```python
from build123d import *

# Parameters (mm, degrees)
SKETCH1_W           = 120
SKETCH1_H           = 140
BOSS_EXTRUDE1_DEPTH = 3
SKETCH2_R           = 1.525
CUT_EXTRUDE1_DEPTH  = 93.244241013
SKETCH3_W           = 10
SKETCH3_H           = 2.05
CUT_EXTRUDE2_DEPTH  = 93.244241013
SKETCH4_R           = 1.5
CUT_EXTRUDE3_DEPTH  = 3
SKETCH5_R           = 1.5
SKETCH5_W           = 50
SKETCH5_H           = 8
CUT_EXTRUDE4_DEPTH  = 3


with BuildPart() as part:
    # Sketch1 → Boss-Extrude1 (new body)
    with BuildSketch(Plane(origin=(0, 0, 0), x_dir=(1, 0, 0), z_dir=(0, 1, 0))):
        Rectangle(SKETCH1_W, SKETCH1_H)
    extrude(amount=BOSS_EXTRUDE1_DEPTH)

    # Sketch2 → Cut-Extrude1 (cut, through all)
    with BuildSketch(Plane(origin=(0, 3, 0), x_dir=(1, 0, 0), z_dir=(0, 1, 0))):
        with Locations(Location((-53, -26.81, 0), (0, 0, 270))):
            Circle(SKETCH2_R)
        with Locations(Location((-54, 60, 0), (0, 0, 270))):
            Circle(SKETCH2_R)
        with Locations(Location((53, -26.81, 0), (0, 0, 90))):
            Circle(SKETCH2_R)
        with Locations(Location((54, 60, 0), (0, 0, 90))):
            Circle(SKETCH2_R)
    extrude(amount=-CUT_EXTRUDE1_DEPTH, mode=Mode.SUBTRACT)

    # Sketch3 → Cut-Extrude2 (cut, through all)
    with BuildSketch(Plane(origin=(0, 3, 0), x_dir=(1, 0, 0), z_dir=(0, 1, 0))):
        with Locations((0, 16.115)):
            Rectangle(SKETCH3_W, SKETCH3_H)
        with Locations((0, -15.985)):
            Rectangle(SKETCH3_W, SKETCH3_H)
        with Locations((0, 61.215)):
            Rectangle(SKETCH3_W, SKETCH3_H)
    extrude(amount=-CUT_EXTRUDE2_DEPTH, mode=Mode.SUBTRACT)

    # Sketch4 → Cut-Extrude3 (cut)
    with BuildSketch(Plane(origin=(0, 3, 0), x_dir=(1, 0, 0), z_dir=(0, 1, 0))):
        with Locations(Location((-52, -50, 0), (0, 0, 270))):
            Circle(SKETCH4_R)
        with Locations(Location((-45.815341562, -62, 0), (0, 0, 270))):
            Circle(SKETCH4_R)
        with Locations(Location((45.815341562, -62, 0), (0, 0, 90))):
            Circle(SKETCH4_R)
        with Locations(Location((52, -50, 0), (0, 0, 90))):
            Circle(SKETCH4_R)
    extrude(amount=-CUT_EXTRUDE3_DEPTH, mode=Mode.SUBTRACT)

    # Sketch5 → Cut-Extrude4 (cut)
    with BuildSketch(Plane(origin=(0, 3, 0), x_dir=(1, 0, 0), z_dir=(0, 1, 0))):
        with Locations(Location((-36.8, -65, 0), (0, 0, 270))):
            Circle(SKETCH5_R)
        with Locations(Location((36.8, -65, 0), (0, 0, 90))):
            Circle(SKETCH5_R)
        with Locations((0, -55.5)):
            Rectangle(SKETCH5_W, SKETCH5_H)
    extrude(amount=-CUT_EXTRUDE4_DEPTH, mode=Mode.SUBTRACT)


solid = part.part
```
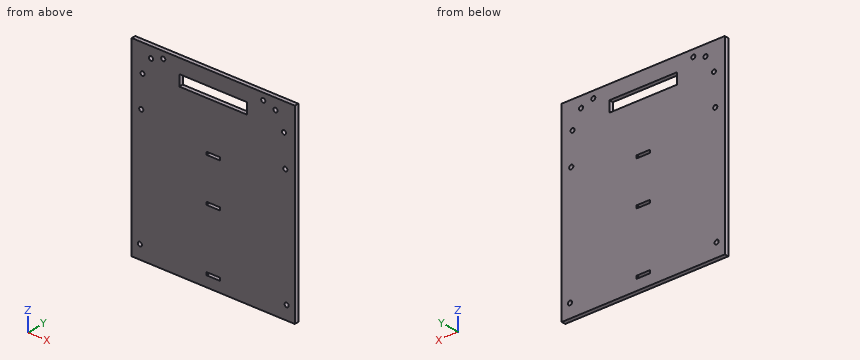
CAD build for the part. Positions are in the model's coordinates, mm. Round coordinates to 2 decimals unless told otherwise and drop trailing zeros. Write each loop counter-clockwise with the first axis right and the second up, starting at its lowest first coordinate (ties: lowest second). Pieces come first, ordered by that corner, then holes. Notation, with made-up numbers: (18.5, 61) -> (72.5, 61) arc R9 cw to (72.5, 68) -> close; hole circle Ø2 at (6.25, -25.75). An arc over 180 degrees is marked (long way). Answer in a Markdown table with one row per item. Add a question column.
Item 1: Saw through at A-A, the plane z = 62. Write the cut outline in (x, y), then the cut area to 3 significant figures.
Item 2: Saw through at B-B, the plane x = 36.8. Write the cut outline in (y, z).
Item 3: Drill centre lines: line 1 (X direction, y = 2.25, z = 65); line 2 (X direction, y = 1.25, z = -60) (3 decimals); line 3 (Z direction, x = -24.5, y = 2.5). Where is each one in solid material? Low to high. Write a range as from..to.
Item 4: Saw through at C-C, the plane y = 0.85. Count the separate pieces of the cut face and the enclosed holes in it, then the cut area to 3 significant figures.
Findings below:
| question | item | result |
|---|---|---|
| 1 | outline | (-60, 0) -> (-47.32, 0) -> (-47.32, 3) -> (-60, 3) -> close; (-44.32, 0) -> (44.32, 0) -> (44.32, 3) -> (-44.32, 3) -> close; (47.32, 0) -> (60, 0) -> (60, 3) -> (47.32, 3) -> close |
| 1 | area | 342 mm^2 |
| 2 | outline | (0, -70) -> (3, -70) -> (3, 63.5) -> (0, 63.5) -> close; (0, 66.5) -> (3, 66.5) -> (3, 70) -> (0, 70) -> close |
| 3 | line 1 | x = -60..-38.3, -35.3..35.3, 38.3..60 |
| 3 | line 2 | x = -60..-55.525, -52.475..52.475, 55.525..60 |
| 3 | line 3 | z = -70..51.5, 59.5..70 |
| 4 | separate pieces | 1 |
| 4 | enclosed holes | 14 |
| 4 | area | 16,300 mm^2 |
